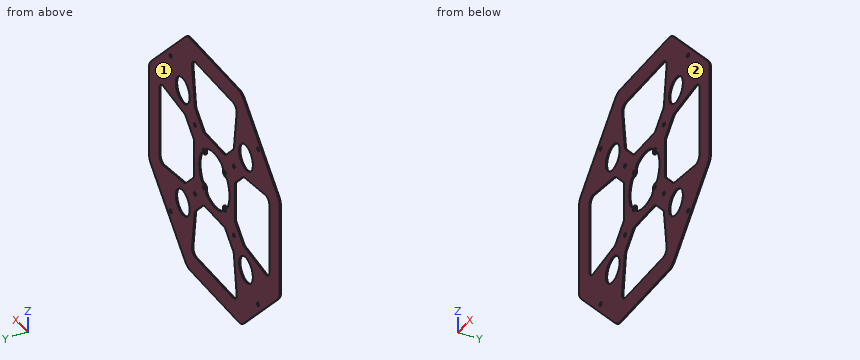
from build123d import *

# Parameters (mm, degrees)
SKETCH1_R           = 1.5
SKETCH1_R_2         = 10
BOSS_EXTRUDE1_DEPTH = 1


with BuildPart() as part:
    # Sketch1 → Boss-Extrude1 (new body)
    with BuildSketch(Plane(origin=(0, 0, 0), x_dir=(1, 0, 0), z_dir=(0, 1, 0))):
        with BuildLine():
            Line((92.071067812, 42.279220614), (42.279220614, 92.071067812))
            ThreePointArc((42.279220614, 92.071067812), (39.034987125, 94.238795325), (35.208152802, 95))
            Line((35.208152802, 95), (-35.208152802, 95))
            ThreePointArc((-35.208152802, 95), (-39.034987125, 94.238795325), (-42.279220614, 92.071067812))
            Line((-42.279220614, 92.071067812), (-92.071067812, 42.279220614))
            ThreePointArc((-92.071067812, 42.279220614), (-94.238795325, 39.034987125), (-95, 35.208152802))
            Line((-95, 35.208152802), (-95, -35.208152802))
            ThreePointArc((-95, -35.208152802), (-94.238795325, -39.034987125), (-92.071067812, -42.279220614))
            Line((-92.071067812, -42.279220614), (-42.279220614, -92.071067812))
            ThreePointArc((-42.279220614, -92.071067812), (-39.034987125, -94.238795325), (-35.208152802, -95))
            Line((-35.208152802, -95), (35.208152802, -95))
            ThreePointArc((35.208152802, -95), (39.034987125, -94.238795325), (42.279220614, -92.071067812))
            Line((42.279220614, -92.071067812), (92.071067812, -42.279220614))
            ThreePointArc((92.071067812, -42.279220614), (94.238795325, -39.034987125), (95, -35.208152802))
            Line((95, -35.208152802), (95, 35.208152802))
            ThreePointArc((95, 35.208152802), (94.238795325, 39.034987125), (92.071067812, 42.279220614))
        make_face()
        with Locations(Location((63.639610307, 63.639610307, 0), (0, 0, 270))):
            Circle(SKETCH1_R, mode=Mode.SUBTRACT)
        with Locations(Location((28.284271247, 28.284271247, 0), (0, 0, 270))):
            Circle(SKETCH1_R, mode=Mode.SUBTRACT)
        with Locations(Location((63.639610307, -63.639610307, 0), (0, 0, 270))):
            Circle(SKETCH1_R, mode=Mode.SUBTRACT)
        with Locations(Location((28.284271247, -28.284271247, 0), (0, 0, 270))):
            Circle(SKETCH1_R, mode=Mode.SUBTRACT)
        with Locations(Location((-63.639610307, -63.639610307, 0), (0, 0, 270))):
            Circle(SKETCH1_R, mode=Mode.SUBTRACT)
        with Locations(Location((-28.284271247, -28.284271247, 0), (0, 0, 270))):
            Circle(SKETCH1_R, mode=Mode.SUBTRACT)
        with Locations(Location((-63.639610307, 63.639610307, 0), (0, 0, 270))):
            Circle(SKETCH1_R, mode=Mode.SUBTRACT)
        with Locations(Location((-28.284271247, 28.284271247, 0), (0, 0, 270))):
            Circle(SKETCH1_R, mode=Mode.SUBTRACT)
        with Locations(Location((-45.961940777, 45.961940777, 0), (0, 0, 270))):
            Circle(SKETCH1_R_2, mode=Mode.SUBTRACT)
        with Locations(Location((45.961940777, 45.961940777, 0), (0, 0, 270))):
            Circle(SKETCH1_R_2, mode=Mode.SUBTRACT)
        with Locations(Location((45.961940777, -45.961940777, 0), (0, 0, 270))):
            Circle(SKETCH1_R_2, mode=Mode.SUBTRACT)
        with Locations(Location((-45.961940777, -45.961940777, 0), (0, 0, 270))):
            Circle(SKETCH1_R_2, mode=Mode.SUBTRACT)
        with Locations(Location((15.25, 15.25, 0), (0, 0, 270))):
            Circle(SKETCH1_R, mode=Mode.SUBTRACT)
        with Locations(Location((15.25, -15.25, 0), (0, 0, 270))):
            Circle(SKETCH1_R, mode=Mode.SUBTRACT)
        with Locations(Location((-15.25, -15.25, 0), (0, 0, 270))):
            Circle(SKETCH1_R, mode=Mode.SUBTRACT)
        with Locations(Location((-15.25, 15.25, 0), (0, 0, 270))):
            Circle(SKETCH1_R, mode=Mode.SUBTRACT)
        with BuildLine():
            Line((27.079275596, 41.221411219), (16.142135624, 30.284271247))
            ThreePointArc((16.142135624, 30.284271247), (15.493288926, 29.850725745), (14.727922061, 29.69848481))
            Line((14.727922061, 29.69848481), (-14.727922061, 29.69848481))
            ThreePointArc((-14.727922061, 29.69848481), (-15.493288926, 29.850725745), (-16.142135624, 30.284271247))
            Line((-16.142135624, 30.284271247), (-27.079275596, 41.221411219))
            ThreePointArc((-27.079275596, 41.221411219), (-28.030817483, 42.551009763), (-28.502553799, 44.116490233))
            Line((-28.502553799, 44.116490233), (-32.40859259, 74.359545108))
            ThreePointArc((-32.40859259, 74.359545108), (-31.204928579, 78.301342571), (-27.449780482, 80))
            Line((-27.449780482, 80), (27.449780482, 80))
            ThreePointArc((27.449780482, 80), (31.204928579, 78.301342571), (32.40859259, 74.359545108))
            Line((32.40859259, 74.359545108), (28.502553799, 44.116490233))
            ThreePointArc((28.502553799, 44.116490233), (28.030817483, 42.551009763), (27.079275596, 41.221411219))
        make_face(mode=Mode.SUBTRACT)
        with BuildLine():
            Line((30.284271247, 16.142135624), (41.221411219, 27.079275596))
            ThreePointArc((41.221411219, 27.079275596), (42.551009763, 28.030817483), (44.116490233, 28.502553799))
            Line((44.116490233, 28.502553799), (74.359545108, 32.40859259))
            ThreePointArc((74.359545108, 32.40859259), (78.301342571, 31.204928579), (80, 27.449780482))
            Line((80, 27.449780482), (80, -27.449780482))
            ThreePointArc((80, -27.449780482), (78.301342571, -31.204928579), (74.359545108, -32.40859259))
            Line((74.359545108, -32.40859259), (44.116490233, -28.502553799))
            ThreePointArc((44.116490233, -28.502553799), (42.551009763, -28.030817483), (41.221411219, -27.079275596))
            Line((41.221411219, -27.079275596), (30.284271247, -16.142135624))
            ThreePointArc((30.284271247, -16.142135624), (29.850725745, -15.493288926), (29.69848481, -14.727922061))
            Line((29.69848481, -14.727922061), (29.69848481, 14.727922061))
            ThreePointArc((29.69848481, 14.727922061), (29.850725745, 15.493288926), (30.284271247, 16.142135624))
        make_face(mode=Mode.SUBTRACT)
        with BuildLine():
            Line((16.142135624, -30.284271247), (27.079275596, -41.221411219))
            ThreePointArc((27.079275596, -41.221411219), (28.030817483, -42.551009763), (28.502553799, -44.116490233))
            Line((28.502553799, -44.116490233), (32.40859259, -74.359545108))
            ThreePointArc((32.40859259, -74.359545108), (31.204928579, -78.301342571), (27.449780482, -80))
            Line((27.449780482, -80), (-27.449780482, -80))
            ThreePointArc((-27.449780482, -80), (-31.204928579, -78.301342571), (-32.40859259, -74.359545108))
            Line((-32.40859259, -74.359545108), (-28.502553799, -44.116490233))
            ThreePointArc((-28.502553799, -44.116490233), (-28.030817483, -42.551009763), (-27.079275596, -41.221411219))
            Line((-27.079275596, -41.221411219), (-16.142135624, -30.284271247))
            ThreePointArc((-16.142135624, -30.284271247), (-15.493288926, -29.850725745), (-14.727922061, -29.69848481))
            Line((-14.727922061, -29.69848481), (14.727922061, -29.69848481))
            ThreePointArc((14.727922061, -29.69848481), (15.493288926, -29.850725745), (16.142135624, -30.284271247))
        make_face(mode=Mode.SUBTRACT)
        with BuildLine():
            Line((-30.284271247, -16.142135624), (-41.221411219, -27.079275596))
            ThreePointArc((-41.221411219, -27.079275596), (-42.551009763, -28.030817483), (-44.116490233, -28.502553799))
            Line((-44.116490233, -28.502553799), (-74.359545108, -32.40859259))
            ThreePointArc((-74.359545108, -32.40859259), (-78.301342571, -31.204928579), (-80, -27.449780482))
            Line((-80, -27.449780482), (-80, 27.449780482))
            ThreePointArc((-80, 27.449780482), (-78.301342571, 31.204928579), (-74.359545108, 32.40859259))
            Line((-74.359545108, 32.40859259), (-44.116490233, 28.502553799))
            ThreePointArc((-44.116490233, 28.502553799), (-42.551009763, 28.030817483), (-41.221411219, 27.079275596))
            Line((-41.221411219, 27.079275596), (-30.284271247, 16.142135624))
            ThreePointArc((-30.284271247, 16.142135624), (-29.850725745, 15.493288926), (-29.69848481, 14.727922061))
            Line((-29.69848481, 14.727922061), (-29.69848481, -14.727922061))
            ThreePointArc((-29.69848481, -14.727922061), (-29.850725745, -15.493288926), (-30.284271247, -16.142135624))
        make_face(mode=Mode.SUBTRACT)
        with BuildLine():
            ThreePointArc((22, 0), (21.269941811, -5.620460422), (19.128220423, -10.86789692))
            ThreePointArc((19.128220423, -10.86789692), (17.744295436, -12.124647251), (15.884913364, -12.317955488))
            ThreePointArc((15.884913364, -12.317955488), (13.128679656, -13.128679656), (12.317955488, -15.884913364))
            ThreePointArc((12.317955488, -15.884913364), (12.124647251, -17.744295436), (10.86789692, -19.128220423))
            ThreePointArc((10.86789692, -19.128220423), (5.620460422, -21.269941811), (0, -22))
            ThreePointArc((0, -22), (-5.620460422, -21.269941811), (-10.86789692, -19.128220423))
            ThreePointArc((-10.86789692, -19.128220423), (-12.124647251, -17.744295436), (-12.317955488, -15.884913364))
            ThreePointArc((-12.317955488, -15.884913364), (-13.128679656, -13.128679656), (-15.884913364, -12.317955488))
            ThreePointArc((-15.884913364, -12.317955488), (-17.744295436, -12.124647251), (-19.128220423, -10.86789692))
            ThreePointArc((-19.128220423, -10.86789692), (-21.269941811, -5.620460422), (-22, 0))
            ThreePointArc((-22, 0), (-21.269941811, 5.620460422), (-19.128220423, 10.86789692))
            ThreePointArc((-19.128220423, 10.86789692), (-17.744295436, 12.124647251), (-15.884913364, 12.317955488))
            ThreePointArc((-15.884913364, 12.317955488), (-13.128679656, 13.128679656), (-12.317955488, 15.884913364))
            ThreePointArc((-12.317955488, 15.884913364), (-12.124647251, 17.744295436), (-10.86789692, 19.128220423))
            ThreePointArc((-10.86789692, 19.128220423), (-5.620460422, 21.269941811), (0, 22))
            ThreePointArc((0, 22), (5.620460422, 21.269941811), (10.86789692, 19.128220423))
            ThreePointArc((10.86789692, 19.128220423), (12.124647251, 17.744295436), (12.317955488, 15.884913364))
            ThreePointArc((12.317955488, 15.884913364), (13.128679656, 13.128679656), (15.884913364, 12.317955488))
            ThreePointArc((15.884913364, 12.317955488), (17.744295436, 12.124647251), (19.128220423, 10.86789692))
            ThreePointArc((19.128220423, 10.86789692), (21.269941811, 5.620460422), (22, 0))
        make_face(mode=Mode.SUBTRACT)
    extrude(amount=BOSS_EXTRUDE1_DEPTH)


solid = part.part
Input: part model. Units: mm. Frame: model coordinates. Face numbers are marked on the shaded views. Coordinates: 2 decimals unless noted, no trailing zeros. Loops run counter-clockwise (first coordinate to the right, second up) from the corner with the lowest first, then second, coordinate; pieces in that order, holes last.
Q1. Cut plane C-C (y = 0.4). Give the number of separate pieces and of enclosed holes in the cut face, then the cut area to 3 significant figures.
Q2. Cut plane A-A (z = 39). Output: boundary loops of the cut face in (x, y), then the cut area to 3 significant figures.
Q3. Cut plane B-B (x = 52). Output: boundary loops of the cut face in (y, z), then the cut area to 3 significant figures.
Q4. Contact query for a flat-ended pin moving along its axis: pin 1 (6 mm diameter, centred on x = 31.5, z = 4, fed in from +Y). Output: stop coordinate, or through.
Q5. Material intervals for line 1 (X direction, y = 0.2, z = -15.25); line 2 (X direction, y = 0.8, z = -42.5); line 3 (Z direction, x = 54.5, y = 0.45), sorted ascending.
Q6. Draft query along Y for the marked faces 1 and 2. Return one class per face: +Y half, -Y half, draft (parallel to the pull), parting line (faces both ways), or undercut.
Working result:
1. separate pieces: 1
1. enclosed holes: 21
1. area: 15,700 mm2
2. outline: (-94.25, 0) - (-53.14, 0) - (-53.14, 1) - (-94.25, 1) - close; (-38.78, 0) - (-24.86, 0) - (-24.86, 1) - (-38.78, 1) - close; (24.86, 0) - (38.78, 0) - (38.78, 1) - (24.86, 1) - close; (53.14, 0) - (94.25, 0) - (94.25, 1) - (53.14, 1) - close
2. area: 110 mm2
3. outline: (0, -82.35) - (1, -82.35) - (1, -53.93) - (0, -53.93) - close; (0, -37.99) - (1, -37.99) - (1, -29.52) - (0, -29.52) - close; (0, 29.52) - (1, 29.52) - (1, 37.99) - (0, 37.99) - close; (0, 53.93) - (1, 53.93) - (1, 82.35) - (0, 82.35) - close
3. area: 73.8 mm2
4. pin 1: stops at y = 1
5. line 1: x = -95 to -80, -29.77 to -16.75, -13.75 to -12.25, 12.25 to 13.75, 16.75 to 29.77, 80 to 95
5. line 2: x = -91.85 to -55.34, -36.58 to -28.01, 28.01 to 36.58, 55.34 to 91.85
5. line 3: z = -79.85 to -51.17, -40.76 to -29.84, 29.84 to 40.76, 51.17 to 79.85
6. face 1: +Y half
6. face 2: -Y half
